from build123d import *

# Parameters (mm, degrees)
SKETCH1_R           = 1.475
BOSS_EXTRUDE1_DEPTH = 5


with BuildPart() as part:
    # Sketch1 → Boss-Extrude1 (new body)
    with BuildSketch(Plane.XY):
        Polygon((-13.5, 19), (13.5, 19), (13.5, 15.15), (18.5, 15.15), (18.5, 4.85), (13.5, 4.85), (13.5, 1.475), (11.5, 1.475), (11.5, 2.75), (9, 2.75), (9, 1.475), (8, 1.475), (8, -1.475), (9, -1.475), (9, -2.75), (11.5, -2.75), (11.5, -1.475), (13.5, -1.475), (13.5, -4.85), (18.5, -4.85), (18.5, -15.15), (13.5, -15.15), (13.5, -19), (-13.5, -19), (-13.5, -15.15), (-18.5, -15.15), (-18.5, -4.85), (-13.5, -4.85), (-13.5, -1.475), (-11.5, -1.475), (-11.5, -2.75), (-9, -2.75), (-9, -1.475), (-8, -1.475), (-8, 1.475), (-9, 1.475), (-9, 2.75), (-11.5, 2.75), (-11.5, 1.475), (-13.5, 1.475), (-13.5, 4.85), (-18.5, 4.85), (-18.5, 15.15), (-13.5, 15.15), align=None)
        with Locations((0, 14)):
            Circle(SKETCH1_R, mode=Mode.SUBTRACT)
        with Locations((0, -14)):
            Circle(SKETCH1_R, mode=Mode.SUBTRACT)
    extrude(amount=BOSS_EXTRUDE1_DEPTH)


solid = part.part
Work out the finished part from the listing and answer in its coordinate system (mm). A direction names the side the tool comes from. Round coordinates to 2 decimals unless told otherwise and drop trailing zeros. Loops run counter-clockwise (first coordinate to the right, second up) from the corner with the lowest first, then second, coordinate; pieces in that order, holes last. Notation, with made-up numbers: (54.25, 40.5) - (90.25, 40.5) arc R12 cw to (90.25, 63.5) - close; hole circle Ø5 at (28, -34). An arc over 180 degrees is marked (long way). One line per item, written item: value.
Q1. For faces 4 (the flat face through (-13.5, 3, 2)), 5 (the flat face through (9, -2, 2)), 6 (the flat face through (13, 1.475, 2)), determine the directions among +Z, -Z, +X, -X, +Y, -Y from which every point of the face is accessible in a straight line to the end or side of a thin tool.
Check values:
face 4: +Z, -Z, -X
face 5: +Z, -Z
face 6: +Z, -Z, +X
Q2. Find section C-C on x = 9.5. Give the vertices of the cut face in (y, z), and give its area (4 significant figures).
Check values:
outline: (-19, 0) - (-2.75, 0) - (-2.75, 5) - (-19, 5) - close; (2.75, 0) - (19, 0) - (19, 5) - (2.75, 5) - close
area: 162.5 mm2
Q3. Find section D-D on z = 1.45. State how many separate pieces and enclosed holes the cut face has, and give its area (3 significant figures).
Check values:
separate pieces: 1
enclosed holes: 2
area: 1,170 mm2
Q4. Straight lines are drawn through the part: probe 1 along Y at (x, z) = (0, 2.1) (3 decimals); probe 2 along X at (y, z) = (2, 0.45); probe 3 along Y at (x, z) = (14, 4.7). For each, find the intervals that lie inside material, in ascending order.
Check values:
probe 1: -19 to -15.475, -12.525 to 12.525, 15.475 to 19
probe 2: -13.5 to -11.5, -9 to 9, 11.5 to 13.5
probe 3: -15.15 to -4.85, 4.85 to 15.15
Q5. Find section B-B on y = 14. Give the vertices of the cut face in (x, z) (3 decimals), and give its area (3 significant figures).
Check values:
outline: (-18.5, 0) - (-1.475, 0) - (-1.475, 5) - (-18.5, 5) - close; (1.475, 0) - (18.5, 0) - (18.5, 5) - (1.475, 5) - close
area: 170 mm2
Q6. Each of these flat-tipped pins is pushed along its axis until it touches: pin 1 Ø0.6 at (y, z) = (-2.5, 3.5) entering from -X; pin 2 Ø1.9 at (y, z) = (-17, 2.5) entering from +X; pin 3 Ø1.5 at (x, z) = (-15.5, 2.5) entering from +Y. Where does it stop, or does it pass through?
Check values:
pin 1: x = -13.5
pin 2: x = 13.5
pin 3: y = 15.15
Q7. The mould has two halves that part along Y. Classify faces 1 (the cylindrical face through (0.793, -12.756, 2.465)), 2 (the flat face through (16, 15.15, 2)), 3 (the flat face through (13.5, 17, 2)): +Y half, -Y half, draft (parallel to the pull), parting line (faces both ways), or undercut.
Check values:
face 1: undercut
face 2: +Y half
face 3: draft
Q8. Find section A-A on x = 0. Give the vertices of the cut face in (y, z) (3 decimals).
Check values:
outline: (-19, 0) - (-15.475, 0) - (-15.475, 5) - (-19, 5) - close; (-12.525, 0) - (12.525, 0) - (12.525, 5) - (-12.525, 5) - close; (15.475, 0) - (19, 0) - (19, 5) - (15.475, 5) - close
